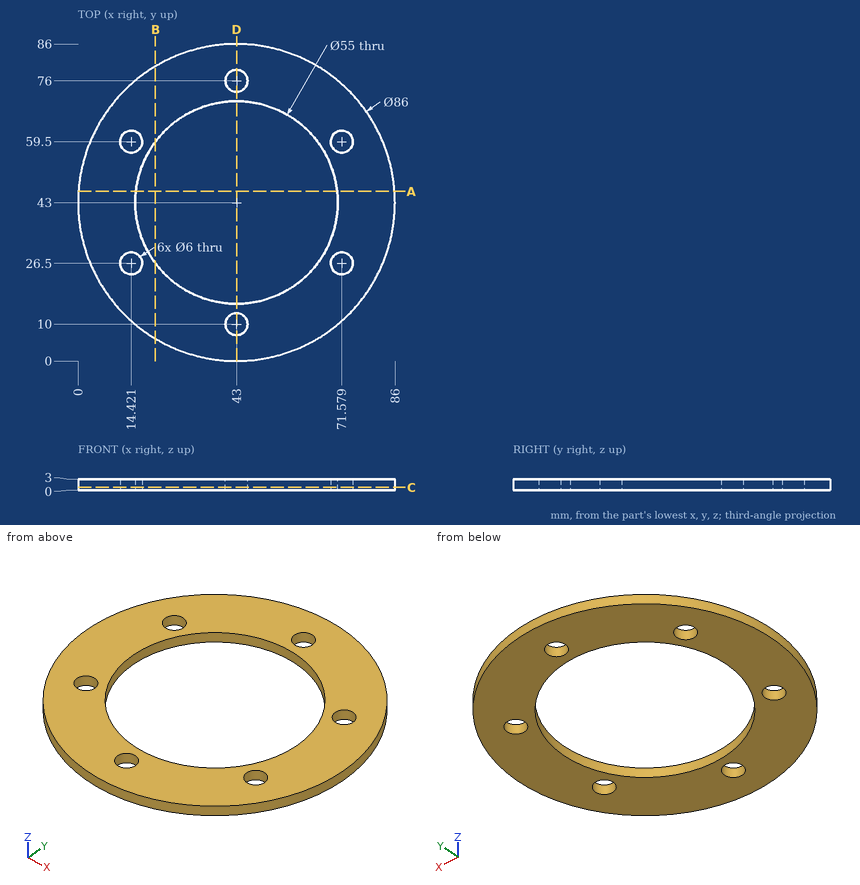
Source: three-view drawing plus pictorial views. Frame: mm from the lowest corner of the part. Give positions to 0.01 mm unless a question says otherwise; leave off trailing zeros. Write each loop counter-clockwise with the first axis right and the second up, starting at its lowest first coordinate (ties: lowest second). Pieces come first, ordered by that corner, then holes.
(1) First-contact query: P1, Ø5, axis at x = 71.58, y = 59.5, coming from the +Z side. Flat tip, straight axial feed; report the tip coordinate or a pass-through.
(2) Cut plane B-B, the plane x = 21. Return loops of the section in (y, z).
(3) Cut plane C-C, the plane z = 0.7. Return loops of the section in (x, y), then the cut area to 3 significant figures.
(4) Ray query, line 1 (Y direction, x = 43, z = 2.1); line 2 (X direction, y = 28.5, z = 0.55) (1 decimal); line 3 (Y direction, x = 45, z = 0.6). Return the intervals inside material, ascending.
(5) Cut plane D-D, the plane x = 43. Return loops of the section in (y, z).
(6) Cut plane A-A, the plane y = 46. Return loops of the section in (x, z) (1 decimal).
Values follow:
1. P1: passes through
2. outline: (6.05, 0) - (26.5, 0) - (26.5, 3) - (6.05, 3) - close; (59.5, 0) - (79.95, 0) - (79.95, 3) - (59.5, 3) - close
3. outline: circle Ø86 at (43, 43); hole circle Ø6 at (14.42, 26.5); hole circle Ø6 at (14.42, 59.5); hole circle Ø55 at (43, 43); hole circle Ø6 at (43, 10); hole circle Ø6 at (43, 76); hole circle Ø6 at (71.58, 26.5); hole circle Ø6 at (71.58, 59.5)
3. area: 3,260 mm2
4. line 1: y = 0 to 7, 13 to 15.5, 70.5 to 73, 79 to 86
4. line 2: x = 2.5 to 12.2, 16.7 to 19.6, 66.4 to 69.3, 73.8 to 83.5
4. line 3: y = 0.05 to 7.76, 12.24 to 15.57, 70.43 to 73.76, 78.24 to 85.95
5. outline: (0, 0) - (7, 0) - (7, 3) - (0, 3) - close; (13, 0) - (15.5, 0) - (15.5, 3) - (13, 3) - close; (70.5, 0) - (73, 0) - (73, 3) - (70.5, 3) - close; (79, 0) - (86, 0) - (86, 3) - (79, 3) - close
6. outline: (0.1, 0) - (15.7, 0) - (15.7, 3) - (0.1, 3) - close; (70.3, 0) - (85.9, 0) - (85.9, 3) - (70.3, 3) - close
